from build123d import *

# Parameters (mm, degrees)
BOSS_EXTRUDE1_DEPTH = 2
CUT_EXTRUDE2_DEPTH  = 1
SKETCH5_R           = 2
CUT_EXTRUDE3_DEPTH  = 21.942838525
CUT_EXTRUDE4_DEPTH  = 21.942838525
SKETCH7_W           = 18.4
SKETCH7_H           = 1
BOSS_EXTRUDE2_DEPTH = 10
SKETCH8_R           = 1.5
CUT_EXTRUDE5_DEPTH  = 25.092211634
CUT_EXTRUDE6_DEPTH  = 1
SKETCH11_W          = 1.421057218
SKETCH11_H          = 17.5
SKETCH11_W_2        = 1.75
SKETCH11_H_2        = 9.84
CUT_EXTRUDE7_DEPTH  = 25.092211634


with BuildPart() as part:
    # Sketch1 → Boss-Extrude1 (new body)
    with BuildSketch(Plane(origin=(0, 0, 0), x_dir=(1, 0, 0), z_dir=(0, 1, 0))):
        with BuildLine():
            Line((-12.649074074, 14.633101852), (5.750925926, 14.633101852))
            ThreePointArc((5.750925926, 14.633101852), (7.377271523, 13.959447449), (8.050925926, 12.333101852))
            Line((8.050925926, 12.333101852), (8.050925926, -6.566898148))
            ThreePointArc((8.050925926, -6.566898148), (7.377271523, -8.193243745), (5.750925926, -8.866898148))
            Line((5.750925926, -8.866898148), (-12.649074074, -8.866898148))
            ThreePointArc((-12.649074074, -8.866898148), (-14.275419671, -8.193243745), (-14.949074074, -6.566898148))
            Line((-14.949074074, -6.566898148), (-14.949074074, 12.333101852))
            ThreePointArc((-14.949074074, 12.333101852), (-14.275419671, 13.959447449), (-12.649074074, 14.633101852))
        make_face()
    extrude(amount=BOSS_EXTRUDE1_DEPTH)

    # Sketch2 → Cut-Extrude2 (cut)
    with BuildSketch(Plane(origin=(0, 2, 0), x_dir=(1, 0, 0), z_dir=(0, 1, 0))):
        with BuildLine():
            Line((5.750925926, 13.633101852), (-12.649074074, 13.633101852))
            ThreePointArc((-12.649074074, 13.633101852), (-13.56831289, 13.252340667), (-13.949074074, 12.333101852))
            Line((-13.949074074, 12.333101852), (-13.949074074, -6.566898148))
            ThreePointArc((-13.949074074, -6.566898148), (-13.56831289, -7.486136964), (-12.649074074, -7.866898148))
            Line((-12.649074074, -7.866898148), (5.750925926, -7.866898148))
            ThreePointArc((5.750925926, -7.866898148), (6.670164741, -7.486136964), (7.050925926, -6.566898148))
            Line((7.050925926, -6.566898148), (7.050925926, 12.333101852))
            ThreePointArc((7.050925926, 12.333101852), (6.670164741, 13.252340667), (5.750925926, 13.633101852))
        make_face()
    extrude(amount=-CUT_EXTRUDE2_DEPTH, mode=Mode.SUBTRACT)

    # Sketch5 → Cut-Extrude3 (cut, through all)
    with BuildSketch(Plane(origin=(0, 1, 0), x_dir=(1, 0, 0), z_dir=(0, 1, 0))):
        with Locations(Location((5.050925926, 11.633101852, 0), (0, 0, 270))):
            Circle(SKETCH5_R)
        with Locations(Location((5.050925926, -5.866898148, 0), (0, 0, 270))):
            Circle(SKETCH5_R)
        with Locations(Location((-11.949074074, -5.866898148, 0), (0, 0, 270))):
            Circle(SKETCH5_R)
        with Locations(Location((-11.949074074, 11.633101852, 0), (0, 0, 90))):
            Circle(SKETCH5_R)
    extrude(amount=-CUT_EXTRUDE3_DEPTH, mode=Mode.SUBTRACT)

    # Sketch6 → Cut-Extrude4 (cut, through all)
    with BuildSketch(Plane(origin=(0, 1, 0), x_dir=(1, 0, 0), z_dir=(0, 1, 0))):
        with BuildLine():
            Line((4.050925926, -3.038471023), (4.050925926, 8.804674727))
            ThreePointArc((4.050925926, 8.804674727), (2.601436183, 9.901051044), (2.050925926, 11.633101852))
            Line((2.050925926, 11.633101852), (2.050925926, -5.866898148))
            ThreePointArc((2.050925926, -5.866898148), (2.601436183, -4.134847341), (4.050925926, -3.038471023))
        make_face()
        with BuildLine():
            Line((-10.949074074, 8.804674727), (-10.949074074, -3.038471023))
            ThreePointArc((-10.949074074, -3.038471023), (-9.499584331, -4.134847341), (-8.949074074, -5.866898148))
            Line((-8.949074074, -5.866898148), (-8.949074074, 11.633101852))
            ThreePointArc((-8.949074074, 11.633101852), (-9.499584331, 9.901051044), (-10.949074074, 8.804674727))
        make_face()
    extrude(amount=-CUT_EXTRUDE4_DEPTH, mode=Mode.SUBTRACT)

    # Sketch7 → Boss-Extrude2 (add)
    with BuildSketch(Plane.XY.offset(8.866898148)):
        with Locations((-3.449074074, 0.5)):
            Rectangle(SKETCH7_W, SKETCH7_H)
    extrude(amount=BOSS_EXTRUDE2_DEPTH)

    # Sketch8 → Cut-Extrude5 (cut, through all)
    with BuildSketch(Plane(origin=(0, 1, 0), x_dir=(1, 0, 0), z_dir=(0, 1, 0))):
        with Locations(Location((1.150925926, -13.866898148, 0), (0, 0, 270))):
            Circle(SKETCH8_R)
        with Locations(Location((-8.049074074, -13.866898148, 0), (0, 0, 270))):
            Circle(SKETCH8_R)
    extrude(amount=-CUT_EXTRUDE5_DEPTH, mode=Mode.SUBTRACT)

    # Sketch9 → Cut-Extrude6 (cut)
    with BuildSketch(Plane(origin=(0, 2, 0), x_dir=(1, 0, 0), z_dir=(0, 1, 0))):
        with BuildLine():
            Line((5.750925926, 13.833101852), (-12.649074074, 13.833101852))
            ThreePointArc((-12.649074074, 13.833101852), (-13.709734246, 13.393762024), (-14.149074074, 12.333101852))
            Line((-14.149074074, 12.333101852), (-14.149074074, -6.566898148))
            ThreePointArc((-14.149074074, -6.566898148), (-13.709734246, -7.62755832), (-12.649074074, -8.066898148))
            Line((-12.649074074, -8.066898148), (5.750925926, -8.066898148))
            ThreePointArc((5.750925926, -8.066898148), (6.811586098, -7.62755832), (7.250925926, -6.566898148))
            Line((7.250925926, -6.566898148), (7.250925926, 12.333101852))
            ThreePointArc((7.250925926, 12.333101852), (6.811586098, 13.393762024), (5.750925926, 13.833101852))
        make_face()
    extrude(amount=-CUT_EXTRUDE6_DEPTH, mode=Mode.SUBTRACT)

    # Sketch11 → Cut-Extrude7 (cut, through all)
    with BuildSketch(Plane(origin=(0, 1, 0), x_dir=(1, 0, 0), z_dir=(0, 1, 0))):
        with Locations((-8.238545465, 2.883101852)):
            Rectangle(SKETCH11_W, SKETCH11_H)
        with Locations((1.340397317, 2.883101852)):
            Rectangle(SKETCH11_W, SKETCH11_H)
        with Locations((-11.824074074, 2.883101852)):
            Rectangle(SKETCH11_W_2, SKETCH11_H_2)
        with Locations((4.925925926, 2.883101852)):
            Rectangle(SKETCH11_W_2, SKETCH11_H_2)
    extrude(amount=-CUT_EXTRUDE7_DEPTH, mode=Mode.SUBTRACT)


solid = part.part
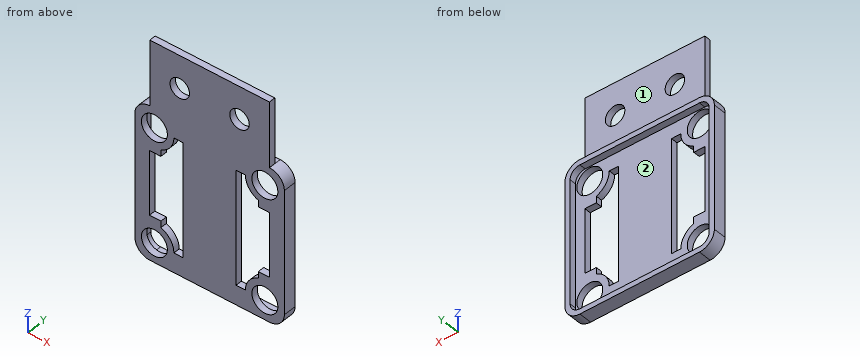
Work out the finished part from the listing and answer in its coordinate system (mm). Face numbers are marked on the shaded views. Coordinates: 2 decimals unless noted, no trailing zeros. Write each loop counter-clockwise with the first axis right and the second up, starting at its lowest first coordinate (ties: lowest second). Pieces come first, ordered by that corner, then holes. Notation, with made-up numbers: M 6.5,-38 L 56.5,-38 A14 ccw 56.5,-20 Z; hole C 27.5,30 d7. An arc over 180 degrees is marked long. Answer as CSV lines item,"result". Start each with the question number.
Item 1: Determine the mould class of the marked faces 1 and 2 for opening direction Z: released by +Z, released by -Z, zero draft, split by the parting line, or undercut.
Item 2: Section D-D on z = 5.5 is taken. Write down the section's boundary in (x, y), and give its area (3 significant figures).
Item 3: Section A-A on z = -2 is taken. Write down the section's boundary in (x, y).
Item 4: Section C-C on y = 1.3 is taken. Write down the section's boundary in (x, z).
Item 5: Flat-ended cylindrical pins translate along their axes: P1, Ø6.5, axis at x = -11.95, z = 5.87, coming from the +Y side; P2, Ø0.5, axis at x = -1.5, y = 1.5, coming from the +Z side; P3, Ø6, axis at x = -5.5, z = -4, coming from the +Y side. Find the tip coordinate at first contact, or state that the pin passes through.
Item 6: Section B-B on x = -8.5 is taken. Write down the section's boundary in (y, z).
Item 7: Consider L1, parallel to Z at x = -8, y = 0.9; L2, parallel to X at y = 1.75, z = 2.5; L3, parallel to X at y = 0.3, z = -7.5. Determine where each line is inside the solid, lowest interval first.
Checks:
1,face 1,"zero draft"
1,face 2,"undercut"
2,outline,"M -14.95,0 L -13.92,0 L -13.92,1 L -14.15,1 L -14.15,2 L -14.95,2 Z; M -9.98,0 L -8.97,0 L -8.97,1 L -9.98,1 Z; M -7.53,0 L 0.63,0 L 0.63,1 L -7.53,1 Z; M 2.07,0 L 3.08,0 L 3.08,1 L 2.07,1 Z; M 7.02,0 L 8.05,0 L 8.05,2 L 7.25,2 L 7.25,1 L 7.02,1 Z"
2,area,"13.8 mm²"
3,outline,"M -14.95,0 L -12.7,0 L -12.7,1 L -14.15,1 L -14.15,2 L -14.95,2 Z; M -7.53,0 L 0.63,0 L 0.63,1 L -7.53,1 Z; M 5.8,0 L 8.05,0 L 8.05,2 L 7.25,2 L 7.25,1 L 5.8,1 Z"
4,outline,"M -14.95,-12.33 A2.3 ccw -12.65,-14.63 L 5.75,-14.63 A2.3 ccw 8.05,-12.33 L 8.05,6.57 A2.3 ccw 5.75,8.87 L -12.65,8.87 A2.3 ccw -14.95,6.57 Z; hole M -14.15,-12.33 A1.5 ccw -12.65,-13.83 L 5.75,-13.83 A1.5 ccw 7.25,-12.33 L 7.25,6.57 A1.5 ccw 5.75,8.07 L -12.65,8.07 A1.5 ccw -14.15,6.57 Z"
5,P1,"stops at y = 2"
5,P2,"stops at z = 8.87"
5,P3,"stops at y = 1"
6,outline,"M 0,-14.63 L 2,-14.63 L 2,-13.83 L 1,-13.83 L 1,-11.63 L 0,-11.63 Z; M 0,5.87 L 1,5.87 L 1,8.07 L 2,8.07 L 2,8.87 L 1,8.87 L 1,12.44 L 0,12.44 Z; M 0,15.3 L 1,15.3 L 1,18.87 L 0,18.87 Z"
7,L1,"z = -14.63 to -11.63, 5.87 to 12.37, 15.37 to 18.87"
7,L2,"x = -14.95 to -14.15, 7.25 to 8.05"
7,L3,"x = -14.95 to -12.7, -7.53 to 0.63, 5.8 to 8.05"
